Design review of the part shown in the three views and the two pictorial views. Dimensions are in mm from the part's minimum x, y and z. Round coordinates to 2 decimals unless told otherwise and drop trailing zeros. Loops run counter-clockwise (first coordinate to the right, second up) from the corner with the lowest first, then second, coordinate; pieces in that order, holes last.
1) Take a section at B-B (y = 3.75). State the section outline as (x, z) points (1 decimal).
2) Take a section at D-D (x = 78.5). State the section outline as (y, z) points, then the cut area to 3 significant figures.
3) Insertion check: pin 1 (6 mm diameter, centred on x = 67.5, z = 17.5, fed in from -Y); pin 2 (5 mm diameter, centred on x = 49.403, z = 30.353, fed in from +Y); pin 3 (3 mm diameter, centred on y = 3.5, z = 26.5, fed in from -X); pin 4 (3 mm diameter, centred on y = 3, z = 79, fed in from -X). Each pin has a flat end and moves straight along its axis. Give the tip position at first contact, or say it passes through.
4) Wall thickness on L1, parallel to Z at x = 51, y = 2 (1 decimal); L2, parallel to Z at x = 53, y = 1.25 (1 decimal); L3, parallel to X at y = 4.25, z = 68 (1 decimal): over which ranges is each line inside the solid? List them lowest first.
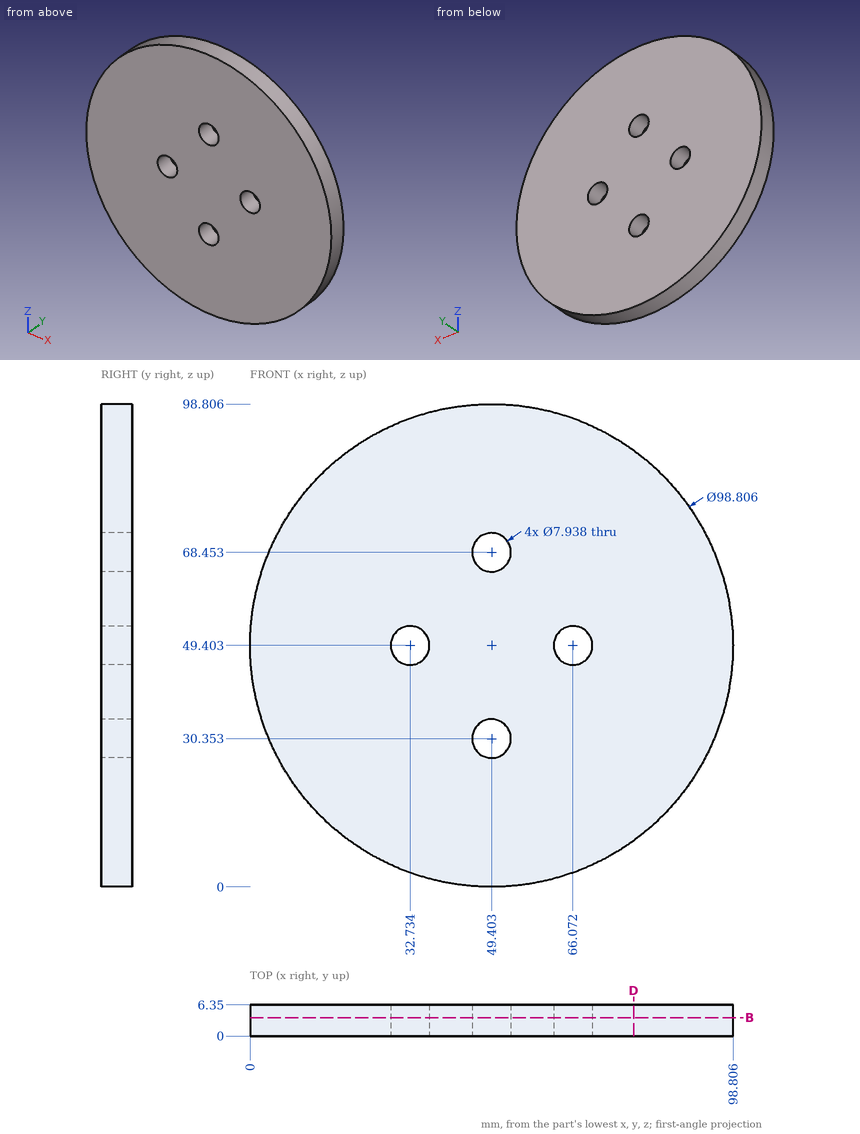
Response:
1. outline: circle Ø98.8 at (49.4, 49.4); hole circle Ø7.9 at (32.7, 49.4); hole circle Ø7.9 at (49.4, 30.4); hole circle Ø7.9 at (49.4, 68.5); hole circle Ø7.9 at (66.1, 49.4)
2. outline: (0, 9.48) - (6.35, 9.48) - (6.35, 89.33) - (0, 89.33) - close
2. area: 507 mm2
3. pin 1: stops at y = 0
3. pin 2: passes through
3. pin 3: stops at x = 4.88
3. pin 4: stops at x = 8.77
4. L1: z = 0 to 26.7, 34 to 64.8, 72.1 to 98.8
4. L2: z = 0.1 to 28.7, 32 to 66.8, 70.1 to 98.7
4. L3: x = 3.6 to 45.5, 53.3 to 95.2
